Can you work these out from the model? Positions are in its coordinate system, mm. A direction names the side the tool comes from. Give positions to 0.01 mm unless a question says otherwise; leave off trailing zeros. Loops run counter-clockwise (first coordinate to the right, second up) from the corner with the lowest first, then second, coordinate; pieces in that order, holes last. Notation, with made-up numbers: M 47.25,46 L 81.25,46 A21 cw 81.25,59 Z; hole C -13,-23.75 d3. An arc over 180 degrees is marked long. Put each result on its own line as item: value. Start each with the question number.
1) For faces 1 (the flat face through (6.09, 1, -41)), 2 (the flat face through (6.09, 1, 2)), 3 (the flat face through (41, 3.55, -19)), 4 (the flat face through (14.5, 1, 2)), 5 (the flat face through (2, 3, -15.295)), which set-ups out of +Z, -Z, +X, -X, +Y, -Y let a thin tool reach every point of the face, with its end or its side?
2) Imagine slicing it at C-C (y = 23). Write out the boundary of the cut face in (x, z) (3 decimals).
3) Imagine slicing it at A-A (y = 18). Write out the boundary of the cut face in (x, z), then the cut area to 3 significant figures.
4) If we mould it in two halves opening along X, with no side actions, what happens to faces 6 (the cylindrical face through (47, 1.3, -19.4)), 7 (the flat face through (18.534, 32.807, -3.317)), 8 (the flat face through (9.5, 3.55, 2.9))? For each: +X half, -X half, draft (parallel to the pull), parting line (faces both ways), or undercut.
5) Imagine slicing it at B-B (z = -40). Write out the boundary of the cut face in (x, y), then the cut area to 3 significant figures.
6) For P1, Ø10, axis at x = 15, y = 10.5, coming from the -Z side; P2, Ø6, axis at y = 7, z = -11.5, coming from the +X side; P3, Ø6, axis at x = 36.5, y = 25, coming from the +Z side, each with a flat end and sliding along its axis, tell me the tip position at first contact or that it passes through.
7) Please list where these lines run through material, in increasing order: line 1 along Z through (x, y) = (32.5, 6.5); line 2 along X through (y, z) = (9, -16.5); line 3 along X through (y, z) = (32, -32). Write a range as from..to.
from build123d import *

# Parameters (mm, degrees)
SKETCH1_W           = 38.59
SKETCH1_H           = 38.59
BOSS_EXTRUDE1_DEPTH = 20.7
SKETCH2_R           = 17.645
BOSS_EXTRUDE2_DEPTH = 12.6
CUT_EXTRUDE1_DEPTH  = 1
SKETCH6_W           = 8
SKETCH6_H           = 4
CUT_EXTRUDE2_DEPTH  = 4
SKETCH8_R           = 4.205
SKETCH8_R_2         = 1.25
BOSS_EXTRUDE3_DEPTH = 3.55
FILLET2_R           = 2
FILLET1_R           = 1


with BuildPart() as part:
    # Sketch1 → Boss-Extrude1 (new body)
    with BuildSketch(Plane(origin=(0, 0, 0), x_dir=(1, 0, 0), z_dir=(0, 1, 0))):
        with Locations((19.295, 19.295)):
            Rectangle(SKETCH1_W, SKETCH1_H)
    extrude(amount=BOSS_EXTRUDE1_DEPTH)

    # Sketch2 → Boss-Extrude2 (add)
    with BuildSketch(Plane(origin=(0, 20.7, 0), x_dir=(1, 0, 0), z_dir=(0, 1, 0))):
        with Locations(Location((19.295, 19.295, 0), (0, 0, 270))):
            Circle(SKETCH2_R)
    extrude(amount=BOSS_EXTRUDE2_DEPTH)

    # Sketch3 → Cut-Extrude1 (cut)
    with BuildSketch(Plane(origin=(0, 33.3, 0), x_dir=(1, 0, 0), z_dir=(0, 1, 0))):
        Polygon((17.795, 4.598076211), (19.295, 2), (20.795, 4.598076211), align=None)
    extrude(amount=-CUT_EXTRUDE1_DEPTH, mode=Mode.SUBTRACT)

    # Sketch6 → Cut-Extrude2 (cut)
    with BuildSketch(Plane(origin=(0, 0, 0), x_dir=(0, 0, -1), z_dir=(1, 0, 0))):
        with Locations((19.295, 3)):
            Rectangle(SKETCH6_W, SKETCH6_H)
    extrude(amount=CUT_EXTRUDE2_DEPTH, mode=Mode.SUBTRACT)

    # Sketch8 → Boss-Extrude3 (add)
    # profile 1 of 9: a face of its own
    with BuildSketch(Plane.XZ):
        with BuildLine():
            ThreePointArc((10.294999977, 0), (7.321615977, 1.231615993), (6.09, 4.205))
            Line((6.09, 4.205), (6.09, 0))
            Line((6.09, 0), (10.294999977, 0))
        make_face()
    # profile 2 of 9: a face of its own
    with BuildSketch(Plane.XZ):
        with BuildLine():
            Line((14.5, 0), (14.5, 4.205))
            ThreePointArc((14.5, 4.205), (13.268384007, 1.231615977), (10.294999977, 0))
            Line((10.294999977, 0), (14.5, 0))
        make_face()
    # profile 3 of 9: a face of its own
    with BuildSketch(Plane.XZ):
        with Locations((10.295, 4.205)):
            Circle(SKETCH8_R)
        with Locations(Location((10.295, 4.205, 0), (0, 0, 270))):
            Circle(SKETCH8_R_2, mode=Mode.SUBTRACT)
    # profile 4 of 9: a face of its own
    with BuildSketch(Plane.XZ):
        with BuildLine():
            Line((42.795, -15.09), (38.59, -15.09))
            Line((38.59, -15.09), (38.59, -19.295))
            ThreePointArc((38.59, -19.295), (39.821615985, -16.321615985), (42.795, -15.09))
        make_face()
    # profile 5 of 9: a face of its own
    with BuildSketch(Plane.XZ):
        with BuildLine():
            ThreePointArc((42.795, -23.5), (39.821615985, -22.268384015), (38.59, -19.295))
            Line((38.59, -19.295), (38.59, -23.5))
            Line((38.59, -23.5), (42.795, -23.5))
        make_face()
    # profile 6 of 9: a face of its own
    with BuildSketch(Plane.XZ):
        with Locations((42.795, -19.295)):
            Circle(SKETCH8_R)
        with Locations(Location((42.795, -19.295, 0), (0, 0, 270))):
            Circle(SKETCH8_R_2, mode=Mode.SUBTRACT)
    # profile 7 of 9: a face of its own
    with BuildSketch(Plane.XZ):
        with BuildLine():
            ThreePointArc((6.09, -42.795), (7.321615985, -39.821615985), (10.295, -38.59))
            Line((10.295, -38.59), (6.09, -38.59))
            Line((6.09, -38.59), (6.09, -42.795))
        make_face()
    # profile 8 of 9: a face of its own
    with BuildSketch(Plane.XZ):
        with Locations((10.295, -42.795)):
            Circle(SKETCH8_R)
        with Locations(Location((10.295, -42.795, 0), (0, 0, 270))):
            Circle(SKETCH8_R_2, mode=Mode.SUBTRACT)
    # profile 9 of 9: a face of its own
    with BuildSketch(Plane.XZ):
        with BuildLine():
            Line((14.5, -42.795), (14.5, -38.59))
            Line((14.5, -38.59), (10.295, -38.59))
            ThreePointArc((10.295, -38.59), (13.268384015, -39.821615985), (14.5, -42.795))
        make_face()
    extrude(amount=-BOSS_EXTRUDE3_DEPTH)

    # Fillet2
    fillet2_edges = [part.edges().sort_by_distance(p)[0] for p in [
        (0, 10.35, -38.59),
        (38.59, 10.35, -38.59),
        (38.59, 10.35, 0),
        (0, 10.35, 0),
    ]]
    fillet(fillet2_edges, radius=FILLET2_R)

    # Fillet1
    # the kernel refuses this fillet: 1 mm, written as the material it takes off along each edge
    with BuildSketch(Plane(origin=(2, 20.7, -36.59), x_dir=(-1, 0, 0), z_dir=(0, 0, 1))) as fillet1_piece_1:
        with BuildLine():
            CenterArc((2 - FILLET1_R, FILLET1_R), FILLET1_R, 270, 90)
            Line((2, FILLET1_R), (2, 0))
            Line((2, 0), (2 - FILLET1_R, 0))
        make_face()
    revolve(axis=Axis((2, 20.7, -36.59), (0, -1, 0)), revolution_arc=90, mode=Mode.SUBTRACT)
    with BuildSketch(Plane(origin=(19.295, 33.3, -19.295), x_dir=(0, 0, 1), z_dir=(-1, 0, 0))) as fillet1_piece_2:
        with BuildLine():
            CenterArc((17.645 - FILLET1_R, -FILLET1_R), FILLET1_R, 0, 90)
            Line((17.645 - FILLET1_R, 0), (17.645, 0))
            Line((17.645, 0), (17.645, -FILLET1_R))
        make_face()
    revolve(axis=Axis((19.295, 33.3, -19.295), (0, 1, 0)), mode=Mode.SUBTRACT)
    with BuildSketch(Plane(origin=(6.09, 3.55, 4.205), x_dir=(0, -1, 0), z_dir=(0, 0, -1)), Plane(origin=(42.795, 3.55, -15.09), x_dir=(0, -1, 0), z_dir=(-1, 0, 0)), Plane(origin=(38.59, 3.55, -23.5), x_dir=(0, -1, 0), z_dir=(1, 0, 0)), Plane(origin=(6.09, 3.55, -38.59), x_dir=(0, -1, 0), z_dir=(0, 0, -1)), Plane(origin=(14.5, 3.55, -42.795), x_dir=(0, -1, 0), z_dir=(0, 0, 1))) as fillet1_piece_3:
        with BuildLine():
            CenterArc((FILLET1_R, -FILLET1_R), FILLET1_R, 90, 90)
            Line((0, -FILLET1_R), (0, 0))
            Line((0, 0), (FILLET1_R, 0))
        make_face()
    extrude(amount=4.205, mode=Mode.SUBTRACT)
    with BuildSketch(Plane(origin=(10.295, 3.55, 4.205), x_dir=(1, 0, 0), z_dir=(0, 0, -1))) as fillet1_piece_4:
        with BuildLine():
            CenterArc((4.205 - FILLET1_R, FILLET1_R), FILLET1_R, 270, 90)
            Line((4.205, FILLET1_R), (4.205, 0))
            Line((4.205, 0), (4.205 - FILLET1_R, 0))
        make_face()
    revolve(axis=Axis((10.295, 3.55, 4.205), (0, -1, 0)), revolution_arc=180, mode=Mode.SUBTRACT)
    with BuildSketch(Plane(origin=(14.5, 3.55, 0), x_dir=(-1, 0, 0), z_dir=(0, 0, 1))) as fillet1_piece_5:
        with BuildLine():
            CenterArc((FILLET1_R, FILLET1_R), FILLET1_R, 180, 90)
            Line((0, FILLET1_R), (0, 0))
            Line((0, 0), (FILLET1_R, 0))
        make_face()
    extrude(amount=4.205, mode=Mode.SUBTRACT)
    with BuildSketch(Plane(origin=(42.795, 3.55, -19.295), x_dir=(0, 0, -1), z_dir=(-1, 0, 0))) as fillet1_piece_6:
        with BuildLine():
            CenterArc((4.205 - FILLET1_R, FILLET1_R), FILLET1_R, 270, 90)
            Line((4.205 - FILLET1_R, 0), (4.205, 0))
            Line((4.205, 0), (4.205, FILLET1_R))
        make_face()
    revolve(axis=Axis((42.795, 3.55, -19.295), (0, -1, 0)), revolution_arc=180, mode=Mode.SUBTRACT)
    with BuildSketch(Plane(origin=(10.295, 3.55, -42.795), x_dir=(-1, 0, 0), z_dir=(0, 0, 1))) as fillet1_piece_7:
        with BuildLine():
            CenterArc((4.205 - FILLET1_R, FILLET1_R), FILLET1_R, 270, 90)
            Line((4.205 - FILLET1_R, 0), (4.205, 0))
            Line((4.205, 0), (4.205, FILLET1_R))
        make_face()
    revolve(axis=Axis((10.295, 3.55, -42.795), (0, -1, 0)), revolution_arc=180, mode=Mode.SUBTRACT)
    with BuildSketch(Plane(origin=(0, 20.7, -36.59), x_dir=(1, 0, 0), z_dir=(0, 0, 1)), Plane(origin=(36.59, 20.7, -38.59), x_dir=(0, 0, 1), z_dir=(-1, 0, 0)), Plane(origin=(38.59, 20.7, -2), x_dir=(-1, 0, 0), z_dir=(0, 0, -1))) as fillet1_piece_8:
        with BuildLine():
            CenterArc((FILLET1_R, -FILLET1_R), FILLET1_R, 90, 90)
            Line((0, -FILLET1_R), (0, 0))
            Line((0, 0), (FILLET1_R, 0))
        make_face()
    extrude(amount=34.59, mode=Mode.SUBTRACT)
    with BuildSketch(Plane(origin=(2, 20.7, 0), x_dir=(0, -1, 0), z_dir=(1, 0, 0))) as fillet1_piece_9:
        with BuildLine():
            CenterArc((FILLET1_R, FILLET1_R), FILLET1_R, 180, 90)
            Line((0, FILLET1_R), (0, 0))
            Line((0, 0), (FILLET1_R, 0))
        make_face()
    extrude(amount=34.59, mode=Mode.SUBTRACT)
    with BuildSketch(Plane(origin=(2, 20.7, -2), x_dir=(0, 0, 1), z_dir=(1, 0, 0))) as fillet1_piece_10:
        with BuildLine():
            CenterArc((2 - FILLET1_R, FILLET1_R), FILLET1_R, 270, 90)
            Line((2 - FILLET1_R, 0), (2, 0))
            Line((2, 0), (2, FILLET1_R))
        make_face()
    revolve(axis=Axis((2, 20.7, -2), (0, -1, 0)), revolution_arc=90, mode=Mode.SUBTRACT)
    with BuildSketch(Plane(origin=(36.59, 20.7, -2), x_dir=(0, 0, 1), z_dir=(-1, 0, 0))) as fillet1_piece_11:
        with BuildLine():
            CenterArc((2 - FILLET1_R, -FILLET1_R), FILLET1_R, 0, 90)
            Line((2, -FILLET1_R), (2, 0))
            Line((2, 0), (2 - FILLET1_R, 0))
        make_face()
    revolve(axis=Axis((36.59, 20.7, -2), (0, 1, 0)), revolution_arc=90, mode=Mode.SUBTRACT)
    with BuildSketch(Plane(origin=(36.59, 20.7, -36.59), x_dir=(1, 0, 0), z_dir=(0, 0, 1))) as fillet1_piece_12:
        with BuildLine():
            CenterArc((2 - FILLET1_R, -FILLET1_R), FILLET1_R, 0, 90)
            Line((2, -FILLET1_R), (2, 0))
            Line((2, 0), (2 - FILLET1_R, 0))
        make_face()
    revolve(axis=Axis((36.59, 20.7, -36.59), (0, 1, 0)), revolution_arc=90, mode=Mode.SUBTRACT)


solid = part.part
Recorded:
1. face 1: -Z, -X, +Y, -Y
1. face 2: +Z, -X, +Y, -Y
1. face 3: +Z, -Z, +X, +Y
1. face 4: +Z, +X, +Y, -Y
1. face 5: -X
2. outline: C 19.295,-19.295 d35.29
3. outline: M 0,-36.59 A2 ccw 2,-38.59 L 36.59,-38.59 A2 ccw 38.59,-36.59 L 38.59,-2 A2 ccw 36.59,0 L 2,0 A2 ccw 0,-2 Z
3. area: 1,490 mm²
4. face 6: +X half
4. face 7: undercut
4. face 8: draft
5. outline: M 6.09,0 L 14.5,0 L 14.5,2.55 A1 ccw 13.5,3.55 L 7.09,3.55 A1 ccw 6.09,2.55 Z
5. area: 29.4 mm²
6. P1: z = -38.59
6. P2: x = 38.59
6. P3: z = -8.83
7. line 1: -38.59..0
7. line 2: 0..38.59
7. line 3: 7.05..31.54
